Study the drawing (mm; zero at the part's minimum x, y, z) and answer. A direction names the side the tool comes from. Give positions to 0.01 mm unless a question says otherwise; leave off trailing zeros. Order: outer loops, then holes, each group sorted by start corner. A loop starts at its lowest first (then second) coordinate and runs counter-clockwise, first axis right, second up. Notation, with made-up numbers: (-18, 58) - (27, 58) arc R29 ccw to (27, 78) - close; hole circle Ø6 at (77.25, -34). An arc over 180 degrees is marked (long way). Put each result on its own line as item: value.
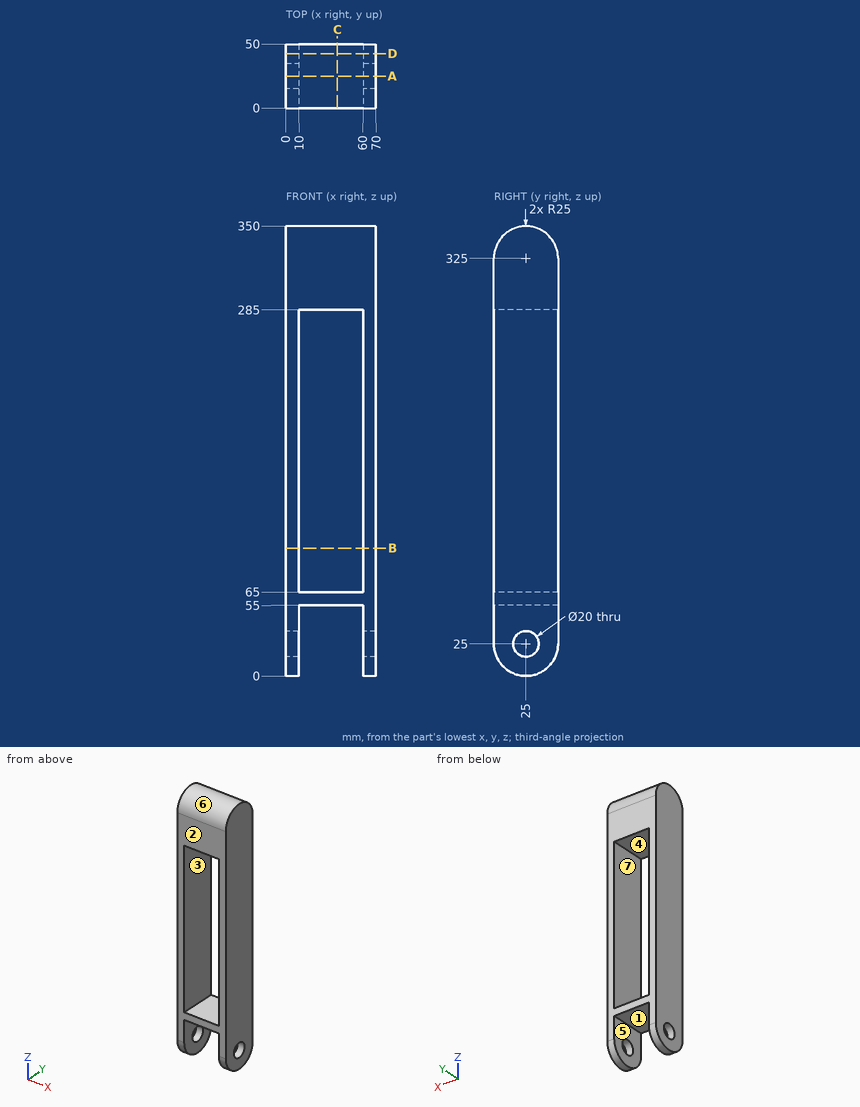
(1) Section B-B, the plane z = 99.5 is taken. Write down the section's boundary in (x, y), then the cut area to 3 significant figures.
Geometry check:
outline: (0, 0) - (10, 0) - (10, 50) - (0, 50) - close; (60, 0) - (70, 0) - (70, 50) - (60, 50) - close
area: 1,000 mm²
(2) Section C-C, the plane x = 40 is taken. Write down the section's boundary in (y, z), then the cut area to 3 significant figures.
Geometry check:
outline: (0, 55) - (50, 55) - (50, 65) - (0, 65) - close; (0, 285) - (50, 285) - (50, 325) arc R25 ccw to (0, 325) - close
area: 3,480 mm²
(3) Given pin 1 (15 mm diameter, centred on y = 15.5, z = 194.5, fed in from -X); pin 2 (10 mm diameter, centred on x = 33.5, y = 12, fed in from +Z); pin 3 (15 mm diameter, centred on x = 32, y = 19, fed in from +Z); pin 4 (15 mm diameter, centred on x = 28, y = 18.5, fed in from -Z), each flat-ended and moving along its own axis, determine where each tip first touches the part or whether it passes through.
Geometry check:
pin 1: stops at x = 0
pin 2: stops at z = 348.69
pin 3: stops at z = 350
pin 4: stops at z = 55
(4) Section D-D, the plane y = 42.5 is taken. Write down the section's boundary in (x, z).
Geometry check:
outline: (0, 7.15) - (10, 7.15) - (10, 55) - (60, 55) - (60, 7.15) - (70, 7.15) - (70, 342.85) - (0, 342.85) - close; hole (10, 65) - (60, 65) - (60, 285) - (10, 285) - close
(5) Determine the mould class of the marked faces 4, 5, 6 and 7 for opening direction Z: pulls with the +Z half, pulls with the -Z half, needs draft (parallel to the pull), parting line crosses it, or undercut.
Geometry check:
face 4: undercut
face 5: needs draft
face 6: pulls with the +Z half
face 7: undercut
(6) Straight lines are drawn through the part: line 1 (X direction, y = 6.5, z = 235.5); line 2 (Z direction, x = 5, y = 25); line 3 (Z direction, x = 28, y = 23.5). For each, find the intervals that lie inside material, in ascending order.
Geometry check:
line 1: x = 0 to 10, 60 to 70
line 2: z = 0 to 15, 35 to 350
line 3: z = 55 to 65, 285 to 349.95
(7) A tool of negligible diameter and unlimited length cuts with its end or side. For the marked faces 1, 2 and 3, from which of +Z, -Z, +X, -X, +Y, -Y can it reach the whole face along a straight path? Write none if from no direction.
Geometry check:
face 1: -Z, +Y, -Y
face 2: +Z, -Z, +X, -X, -Y
face 3: +Y, -Y
(8) Section A-A, the plane y = 25 is taken. Write down the section's boundary in (x, z).
Geometry check:
outline: (0, 0) - (10, 0) - (10, 15) - (0, 15) - close; (0, 35) - (10, 35) - (10, 55) - (60, 55) - (60, 35) - (70, 35) - (70, 350) - (0, 350) - close; (60, 0) - (70, 0) - (70, 15) - (60, 15) - close; hole (10, 65) - (60, 65) - (60, 285) - (10, 285) - close
